```python
from build123d import *

# Parameters (mm, degrees)
BOSS_EXTRUDE1_DEPTH = 1.194
SKETCH2_R           = 0.8065
CUT_EXTRUDE1_DEPTH  = 2.194


with BuildPart() as part:
    # Sketch1 → Boss-Extrude1 (new body)
    with BuildSketch(Plane.XY.offset(2.26)):
        with BuildLine():
            Line((-1.008396957, 3.683), (-19.812, 3.683))
            Line((-19.812, 3.683), (-19.812, -3.683))
            Line((-19.812, -3.683), (19.812, -3.683))
            Line((19.812, -3.683), (19.812, 3.683))
            Line((19.812, 3.683), (1.008396957, 3.683))
            ThreePointArc((1.008396957, 3.683), (0, 3.322929517), (-1.008396957, 3.683))
        make_face()
    extrude(amount=-BOSS_EXTRUDE1_DEPTH)

    # Sketch2 → Cut-Extrude1 (cut, through all)
    with BuildSketch(Plane.XY.offset(2.26)):
        with Locations((-18, -1.885)):
            Circle(SKETCH2_R)
        with Locations((-16.2, 1.885)):
            Circle(SKETCH2_R)
        with Locations((-14.4, -1.885)):
            Circle(SKETCH2_R)
        with Locations((-10.8, -1.885)):
            Circle(SKETCH2_R)
        with Locations((-7.2, -1.885)):
            Circle(SKETCH2_R)
        with Locations((-3.6, -1.885)):
            Circle(SKETCH2_R)
        with Locations((0, -1.885)):
            Circle(SKETCH2_R)
        with Locations((3.6, -1.885)):
            Circle(SKETCH2_R)
        with Locations((7.2, -1.885)):
            Circle(SKETCH2_R)
        with Locations((10.8, -1.885)):
            Circle(SKETCH2_R)
        with Locations((14.4, -1.885)):
            Circle(SKETCH2_R)
        with Locations((18, -1.885)):
            Circle(SKETCH2_R)
        with Locations((-12.6, 1.885)):
            Circle(SKETCH2_R)
        with Locations((-9, 1.885)):
            Circle(SKETCH2_R)
        with Locations((-5.4, 1.885)):
            Circle(SKETCH2_R)
        with Locations((-1.8, 1.885)):
            Circle(SKETCH2_R)
        with Locations((1.8, 1.885)):
            Circle(SKETCH2_R)
        with Locations((5.4, 1.885)):
            Circle(SKETCH2_R)
        with Locations((9, 1.885)):
            Circle(SKETCH2_R)
        with Locations((12.6, 1.885)):
            Circle(SKETCH2_R)
        with Locations((16.2, 1.885)):
            Circle(SKETCH2_R)
    extrude(amount=-CUT_EXTRUDE1_DEPTH, mode=Mode.SUBTRACT)


solid = part.part
```
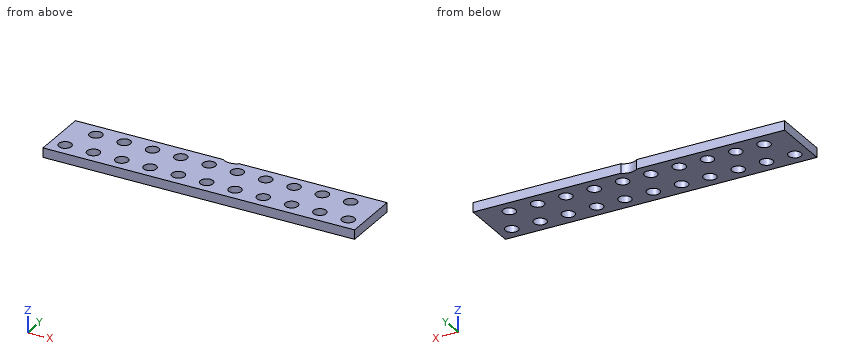
Source: CAD feature listing. Evaluate the final solid. Frame: model axes, mm. Coordinates: 2 decimals unless noted, no trailing zeros. Loops run counter-clockwise (first coordinate to the right, second up) from the corner with the lowest first, then second, coordinate; pieces in that order, holes last. Notation, with made-up numbers: M 9,87.5 L 23,87.5 A25 ccw 23,122.5 Z; hole C 87,76.25 d10. An arc over 180 degrees is marked long. Use a Markdown table: item, result. Add a question column.
Q1. Material intervals for L1, parallel to Y at x = 16.2, z = 1.6; L2, parallel to Y at x = -14.5, z = 1.6; L3, parallel to X at y = 3.5, z = 1.8, sorted ascending.
Q2. Section query C-C, the plane x = 1.5. Return loops of the section in (y, z), and give its area (3 significant figures).
Q3. Section query B-B, the plane z = 1.75. State how many separate pieces and enclosed holes the cut face has, and give its area (3 significant figures).
Q4. Section query A-A, the plane x = -12.6. Return loops of the section in (y, z).
Result:
| question | item | result |
|---|---|---|
| 1 | L1 | y = -3.68 to 1.08, 2.69 to 3.68 |
| 1 | L2 | y = -3.68 to -2.69, -1.08 to 3.68 |
| 1 | L3 | x = -19.81 to -0.73, 0.73 to 19.81 |
| 2 | outline | M -3.68,1.07 L 1.14,1.07 L 1.14,2.26 L -3.68,2.26 Z; M 2.63,1.07 L 3.68,1.07 L 3.68,2.26 L 2.63,2.26 Z |
| 2 | area | 7.01 mm2 |
| 3 | separate pieces | 1 |
| 3 | enclosed holes | 21 |
| 3 | area | 248 mm2 |
| 4 | outline | M -3.68,1.07 L 1.08,1.07 L 1.08,2.26 L -3.68,2.26 Z; M 2.69,1.07 L 3.68,1.07 L 3.68,2.26 L 2.69,2.26 Z |
